Geometry: see drawing. Coordinates: mm, zero at the bounding-box minimum. A direction names the side the tool comes from. Give positions to 0.01 mm unless a question says otherwise; leave off trailing zeros. Write each loop counter-clockwise with the first axis right and the second up, starting at its lowest first coordinate (ties: lowest second). Pieces come first, ordered by that corner, then holes.
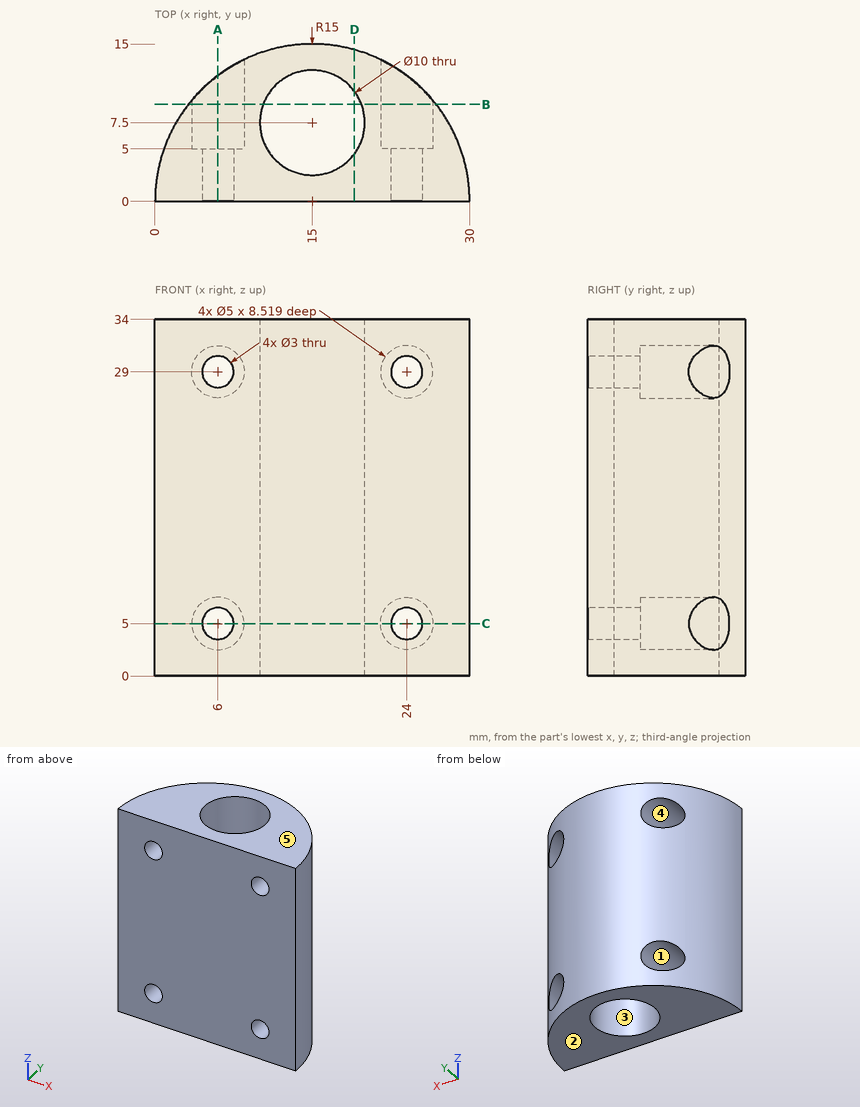
1. Access query for the marked faces 4 and 5. Directions: +Z, -Z, +X, -X, +Y, -Y. A direction counts if a zero-diameter tool reaches every point of the face in a straight line with its end or side. Return the directions, or none.
2. Section query D-D (x = 19). Return loops of the section in (y, z).
3. Section query B-B (y = 9.25). Return loops of the section in (x, z), plus the area to 3 significant figures.
4. Line query: probe 1 along Z at (x, y) = (8, 5.25); probe 2 along X at (y, z) = (2.3, 29); probe 3 along X at (y, z) = (4.75, 21.5) (1 decimal). Output: solid intervals per line, ascending.
5. Pull-direction query (Z, two-part tool) for the marked faces 1, 2 and 3; classes: pulls with the +Z half, pulls with the -Z half, needs draft (parallel to the pull), parting line crosses it, or undercut.
6. Section query A-A (x = 6). Return loops of the section in (y, z), plus the area to 3 significant figures.
7. Pin query (flat end, axial travel): P1, Ø6, axis at y = 13, z = 23.5, coming from the +X side; P2, Ø2.5, axis at x = 6.5, z = 4, coming from the +Y side; P3, Ø2.5, axis at x = 6, z = 5, coming from the +Y side; P4, Ø1.5, axis at x = 14, z = 13, coming from the +Y side. Return the tip coordinate at first contact, or that it passes through.
8. Section query C-C (z = 5). Return loops of the section in (x, y).
The answers:
1. face 4: +Y
1. face 5: +Z, +X, -X, +Y, -Y
2. outline: (0, 0) - (4.5, 0) - (4.5, 34) - (0, 34) - close; (10.5, 0) - (14.46, 0) - (14.46, 34) - (10.5, 34) - close
3. outline: (3.19, 0) - (10.32, 0) - (10.32, 34) - (3.19, 34) - close; (19.68, 0) - (26.81, 0) - (26.81, 34) - (19.68, 34) - close; hole circle Ø5 at (6, 5); hole circle Ø5 at (6, 29); hole circle Ø5 at (24, 5); hole circle Ø5 at (24, 29)
3. area: 406 mm2
4. probe 1: z = 0 to 3.5, 6.5 to 27.5, 30.5 to 34
4. probe 2: x = 0.18 to 4.5, 7.5 to 22.5, 25.5 to 29.82
4. probe 3: x = 0.8 to 10.8, 19.2 to 29.2
5. face 1: undercut
5. face 2: pulls with the -Z half
5. face 3: needs draft
6. outline: (0, 0) - (12, 0) - (12, 2.5) - (5, 2.5) - (5, 3.5) - (0, 3.5) - close; (0, 6.5) - (5, 6.5) - (5, 7.5) - (12, 7.5) - (12, 26.5) - (5, 26.5) - (5, 27.5) - (0, 27.5) - close; (0, 30.5) - (5, 30.5) - (5, 31.5) - (12, 31.5) - (12, 34) - (0, 34) - close
6. area: 308 mm2
7. P1: stops at x = 26.18
7. P2: stops at y = 5
7. P3: passes through
7. P4: stops at y = 15
8. outline: (0, 0) - (4.5, 0) - (4.5, 5) - (3.5, 5) - (3.5, 9.63) arc R15 ccw to start; (7.5, 0) - (22.5, 0) - (22.5, 5) - (21.5, 5) - (21.5, 13.52) arc R15 ccw to (8.5, 13.52) - (8.5, 5) - (7.5, 5) - close; (25.5, 0) - (30, 0) arc R15 ccw to (26.5, 9.63) - (26.5, 5) - (25.5, 5) - close; hole circle Ø10 at (15, 7.5)
